from build123d import *

# Parameters (mm, degrees)
F1_DEPTH = 6.35
F2_R     = 12.7
F2_R_2   = 6.35
F3_DEPTH = 12.7


with BuildPart() as f1:
    # F0 (on Top) → F1 (new body)
    with BuildSketch(Plane.XY):
        with BuildLine():
            Line((44.45, 25.4), (12.7, 25.4))
            ThreePointArc((12.7, 25.4), (0, 12.7), (12.7, 0))
            Line((12.7, 0), (31.75, 0))
            Line((31.75, 0), (44.45, 12.7))
            Line((44.45, 12.7), (44.45, 25.4))
        make_face()
    extrude(amount=F1_DEPTH)

    # F2 (on face) → F3 (join)
    with BuildSketch(Plane.XY.offset(6.35)):
        with Locations((12.7, 12.7)):
            Circle(F2_R)
        with Locations((12.7, 12.7)):
            Circle(F2_R_2, mode=Mode.SUBTRACT)
    extrude(amount=F3_DEPTH)


solid = f1.part
Here's how the part is built. I have some questions about the finished solid (model axes, mm). A direction names the side the tool comes from. Round coordinates to 2 decimals unless told otherwise and drop trailing zeros. Write each loop counter-clockwise with the first axis right and the second up, starting at its lowest first coordinate (ties: lowest second). Pieces come first, ordered by that corner, then holes.
1. If we mould it in two halves opening along X, with no side actions, what happens to faces 3 (the flat face through (44.45, 19, 3)), 4 (the flat face through (32, 13, 6.35)), 5 (the cylindrical face through (8.02, 16.99, 12.61)), 6 (the flat face through (13, 13, 6.35))? For each: released by +X, released by -X, zero draft, split by the parting line, or undercut.
2. Suppose I cut it at A-A (z = 5). List the corners of the cut face in (x, y) for me, and give its area (3 significant figures).
3. Suppose I cut it at B-B (y = 11.5). List the corners of the cut face in (x, z) for me, and give its area (3 significant figures).
4. I need wall thicknesses on L1, parallel to Y at x = 12.7, z = 16; L2, parallel to Z at x = 31, y = 4; L3, parallel to X at y = 15.5, z = 11. Which ranges of each line are inside material? Lowest first, please.
5. For faces 1 (the flat face through (29, 25.4, 3)), 2 (the cylindrical face through (0.012, 13.258, 11.508)), which set-ups out of +Z, -Z, +X, -X, +Y, -Y let a thin tool reach every point of the face, with its end or its side?
6. Will these pins go through, and if not, where does the flat tip stop? pin 1 Ø12.5 at (x, y) = (31.5, 16) entering from +Z; pin 2 Ø8 at (y, z) = (20.5, 2.5) entering from -X; pin 3 Ø2 at (x, z) = (15, 13) entering from +Y.
7. Suppose I cut it at C-C (x = 29.5). List the corners of the cut face in (y, z) for me.
8. Suppose I cut it at D-D (z = 16). List the corners of the cut face in (x, y) for me, and give its area (3 significant figures).
Answer sheet:
1. face 3: released by +X
1. face 4: zero draft
1. face 5: undercut
1. face 6: undercut
2. outline: (12.7, 0) - (31.75, 0) - (44.45, 12.7) - (44.45, 25.4) - (12.7, 25.4) arc R12.7 ccw to start
2. area: 979 mm2
3. outline: (0.06, 0) - (43.25, 0) - (43.25, 6.35) - (25.34, 6.35) - (25.34, 19.05) - (18.94, 19.05) - (18.94, 6.35) - (6.46, 6.35) - (6.46, 19.05) - (0.06, 19.05) - close
3. area: 437 mm2
4. L1: y = 0 to 6.35, 19.05 to 25.4
4. L2: z = 0 to 6.35
4. L3: x = 0.31 to 7, 18.4 to 25.09
5. face 1: +Z, -Z, +X, -X, +Y
5. face 2: +Z
6. pin 1: stops at z = 6.35
6. pin 2: stops at x = 0.58
6. pin 3: stops at y = 25.33
7. outline: (0, 0) - (25.4, 0) - (25.4, 6.35) - (0, 6.35) - close
8. outline: circle Ø25.4 at (12.7, 12.7); hole circle Ø12.7 at (12.7, 12.7)
8. area: 380 mm2
